Could you check a few things on this drawing? It's one solid part, dimensions in mm from its lowest x, y, z. Coordinates: 2 decimals unless noted, no trailing zeros. Write each loop counter-clockwise with the first axis right and the second up, starting at its lowest first coordinate (ties: lowest second). Pieces come first, ordered by that corner, then holes. Notation, with made-up numbers: (20.5, 22) - (28.5, 22) arc R21 cw to (28.5, 37) - close; hole circle Ø11 at (18.5, 18). An arc over 180 degrees is marked (long way). Use one line per item in the form item = value. Start each with the question number.
(1) If we section it at D-D on z = 4.25: Please give me the cut outline in (x, y).
(2) If I drill on probe 1 along X at (y, z) = (55.5, 15.75); probe 2 along X at (y, z) = (60, 16.5) (1 decimal); probe 3 along Y at (x, z) = (66.5, 15.55), over which ranges is the centre line in solid material (lowest first)? Write a range as from..to.
(3) For pin 1 Ø5 at (x, y) = (11.5, 57.5) entering from +Z; pin 2 Ø2 at (y, z) = (71.5, 7.5) entering from -X; pin 3 Ø6 at (y, z) = (20.5, 9) entering from +X; pin 4 Ø20.5 at (x, y) = (47.5, 28.5) entering from +Z, each with a flat end and sliding along its axis, tell me the tip position at first contact or that it passes through.
(4) If we section it at C-C on z = 15.25: Give the number of separate pieces and of enclosed holes in the cut face, then the cut area to 3 significant figures.
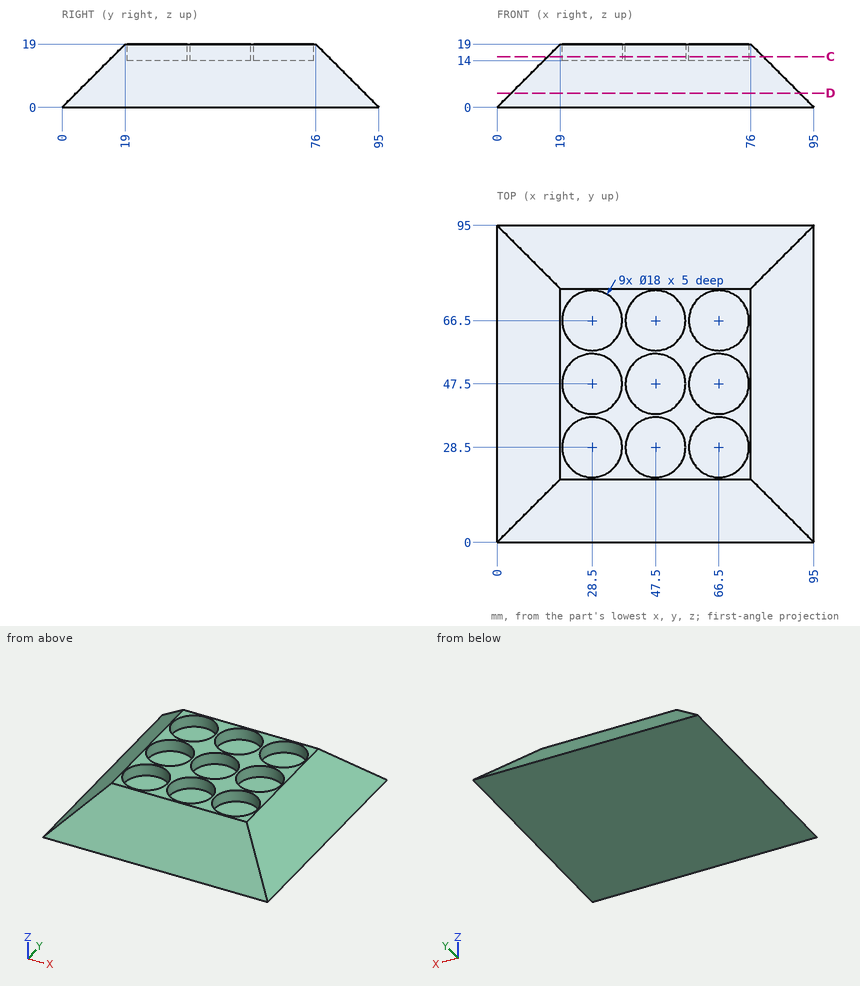
Reported:
q1.outline = (4.25, 4.25) - (90.75, 4.25) - (90.75, 90.75) - (4.25, 90.75) - close
q2.probe_1 = 15.75..24.38, 32.62..43.38, 51.62..62.38, 70.62..79.25
q2.probe_2 = 16.5..22.3, 34.7..41.3, 53.7..60.3, 72.7..78.5
q2.probe_3 = 15.55..19.5, 37.5..38.5, 56.5..57.5, 75.5..79.45
q3.pin_1 = 14
q3.pin_2 = 6.5
q3.pin_3 = 89
q3.pin_4 = 19
q4.separate_pieces = 1
q4.enclosed_holes = 9
q4.area = 1,870 mm2
